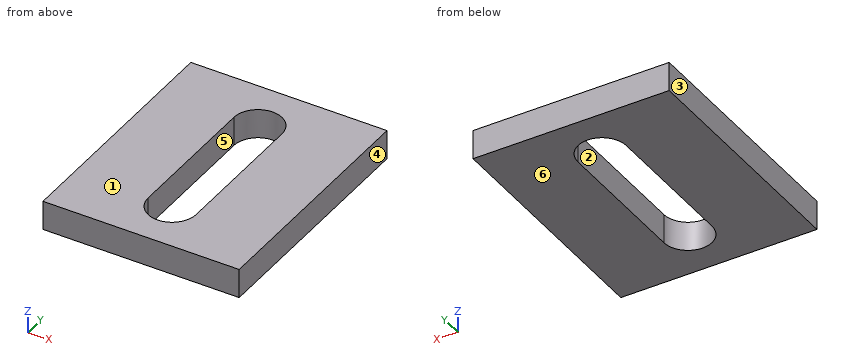
from build123d import *

# Parameters (mm, degrees)
SKETCH_1_W      = 28.812419505
SKETCH_1_H      = 35.7
EXTRUDE_1_DEPTH = 4.3


with BuildPart() as part:
    # 草图1 → 凸台-拉伸1 (new body)
    with BuildSketch(Plane.XY):
        with Locations((17.406209753, -17.85)):
            Rectangle(SKETCH_1_W, SKETCH_1_H)
        with BuildLine():
            ThreePointArc((13.884047379, -28.212407831), (17.406209752, -31.734570205), (20.928372126, -28.212407831))
            Line((20.928372126, -28.212407831), (20.928372126, -7.487592169))
            ThreePointArc((20.928372126, -7.487592169), (17.406209752, -3.965429795), (13.884047379, -7.487592169))
            Line((13.884047379, -7.487592169), (13.884047379, -28.212407831))
        make_face(mode=Mode.SUBTRACT)
    extrude(amount=EXTRUDE_1_DEPTH)


solid = part.part
CAD build for the part. Positions are in the model's coordinates, mm. Face numbers are marked on the shaded views. A direction names the side the tool comes from. Give positions to 0.01 mm unless a question says otherwise; leave off trailing zeros. Write each loop counter-clockwise with the first axis right and the second up, starting at its lowest first coordinate (ties: lowest second). Pieces come first, ordered by that corner, then holes. Notation, with made-up numbers: (-32.75, 43) - (-22.75, 43) arc R14 ccw to (-22.75, 63) - close; hole circle Ø1 at (23.25, 73.25). An arc over 180 degrees is marked (long way). Answer as CSV lines item,"result".
Q1. Drill centre lines: line 1 (X direction, y = -15, z = 0.5); line 2 (X direction, y = -30.5, z = 1.75); line 3 (Y direction, x = 15, z = 0.55). Where is each one in solid material? Low to high. Write a range as from..to.
Result set:
line 1,"3..13.88, 20.93..31.81"
line 2,"3..14.73, 20.08..31.81"
line 3,"-35.7..-30.78, -4.92..0"
Q2. Band-saw the part on C-C (y = -12.5). Give the cut face in (x, z), and give its area (3 significant figures).
Result set:
outline,"(3, 0) - (13.88, 0) - (13.88, 4.3) - (3, 4.3) - close; (20.93, 0) - (31.81, 0) - (31.81, 4.3) - (20.93, 4.3) - close"
area,"93.6 mm²"
Q3. Pull direction X, two halves, no side cores. Call the marked faces 1, 2, 3 and 4: released by +X, released by -X, zero draft, split by the parting line, or undercut.
Result set:
face 1,"zero draft"
face 2,"undercut"
face 3,"released by -X"
face 4,"released by +X"
Q4. 3-axis set-ups, long thin cutter, end or side, ignore diameter. For the marked faces 5 and 6: which of +Z, -Z, +X, -X, +Y, -Y reach the whole face in a straight line?
Result set:
face 5,"+Z, -Z"
face 6,"-Z, +X, -X, +Y, -Y"
Q5. Band-saw the part on B-B (x = 17). Give the cut face in (y, z).
Result set:
outline,"(-35.7, 0) - (-31.71, 0) - (-31.71, 4.3) - (-35.7, 4.3) - close; (-3.99, 0) - (0, 0) - (0, 4.3) - (-3.99, 4.3) - close"
Q6. Band-saw the part on A-A (z = 3.65). Give the cut face in (x, y).
Result set:
outline,"(3, -35.7) - (31.81, -35.7) - (31.81, 0) - (3, 0) - close; hole (13.88, -28.21) arc R3.52 ccw to (20.93, -28.21) - (20.93, -7.49) arc R3.52 ccw to (13.88, -7.49) - close"
